from build123d import *

# Parameters (mm, degrees)
F1_DEPTH = 11
F2_DEPTH = 4


with BuildPart() as f1:
    # F0 (on Top) → F1 (new body)
    with BuildSketch(Plane.XY):
        with BuildLine():
            ThreePointArc((94, 77.5), (93.267767, 79.267767), (91.5, 80))
            Line((91.5, 80), (40.553054, 80))
            Line((40.553054, 80), (23, 80))
            Line((23, 80), (17.5, 80))
            Line((17.5, 80), (-7.5, 80))
            Line((-7.5, 80), (-13, 80))
            Line((-13, 80), (-32.2531, 80))
            Line((-32.2531, 80), (-74.5, 80))
            Line((-74.5, 80), (-91.5, 80))
            ThreePointArc((-91.5, 80), (-93.267767, 79.267767), (-94, 77.5))
            Line((-94, 77.5), (-94, 76))
            Line((-94, 76), (-94, 0))
            Line((-94, 0), (-94, -1.5))
            ThreePointArc((-94, -1.5), (-93.267767, -3.267767), (-91.5, -4))
            Line((-91.5, -4), (-88, -4))
            Line((-88, -4), (88, -4))
            Line((88, -4), (91.5, -4))
            ThreePointArc((91.5, -4), (93.267767, -3.267767), (94, -1.5))
            Line((94, -1.5), (94, 0))
            Line((94, 0), (94, 76))
            Line((94, 76), (94, 77.5))
        make_face()
        with BuildLine():
            ThreePointArc((90, 2.5), (89.267767, 0.732233), (87.5, 0))
            Line((87.5, 0), (-87.5, 0))
            ThreePointArc((-87.5, 0), (-89.267767, 0.732233), (-90, 2.5))
            Line((-90, 2.5), (-90, 73.5))
            ThreePointArc((-90, 73.5), (-89.267767, 75.267767), (-87.5, 76))
            Line((-87.5, 76), (87.5, 76))
            ThreePointArc((87.5, 76), (89.267767, 75.267767), (90, 73.5))
            Line((90, 73.5), (90, 2.5))
        make_face(mode=Mode.SUBTRACT)
    extrude(amount=F1_DEPTH)

    # F0 (on Top) → F2 (join)
    with BuildSketch(Plane.XY):
        with BuildLine():
            Line((-87.5, 0), (87.5, 0))
            ThreePointArc((87.5, 0), (89.267767, 0.732233), (90, 2.5))
            Line((90, 2.5), (90, 73.5))
            ThreePointArc((90, 73.5), (89.267767, 75.267767), (87.5, 76))
            Line((87.5, 76), (-87.5, 76))
            ThreePointArc((-87.5, 76), (-89.267767, 75.267767), (-90, 73.5))
            Line((-90, 73.5), (-90, 2.5))
            ThreePointArc((-90, 2.5), (-89.267767, 0.732233), (-87.5, 0))
        make_face()
        with BuildLine():
            Line((-77.5, 66), (77.5, 66))
            ThreePointArc((77.5, 66), (79.267767, 65.267767), (80, 63.5))
            Line((80, 63.5), (80, 12.5))
            ThreePointArc((80, 12.5), (79.267767, 10.732233), (77.5, 10))
            Line((77.5, 10), (-77.5, 10))
            ThreePointArc((-77.5, 10), (-79.267767, 10.732233), (-80, 12.5))
            Line((-80, 12.5), (-80, 63.5))
            ThreePointArc((-80, 63.5), (-79.267767, 65.267767), (-77.5, 66))
        make_face(mode=Mode.SUBTRACT)
        with BuildLine():
            Line((-32.2531, 80), (-13, 80))
            Line((-13, 80), (-13, 89.5))
            ThreePointArc((-13, 89.5), (-13.732233, 91.267767), (-15.5, 92))
            Line((-15.5, 92), (-29.7531, 92))
            ThreePointArc((-29.7531, 92), (-31.520867, 91.267767), (-32.2531, 89.5))
            Line((-32.2531, 89.5), (-32.2531, 80))
        make_face()
        with BuildLine():
            Line((-7.5, 80), (17.5, 80))
            Line((17.5, 80), (17.5, 89.5))
            ThreePointArc((17.5, 89.5), (16.767767, 91.267767), (15, 92))
            Line((15, 92), (-5, 92))
            ThreePointArc((-5, 92), (-6.767767, 91.267767), (-7.5, 89.5))
            Line((-7.5, 89.5), (-7.5, 80))
        make_face()
        with BuildLine():
            Line((23, 80), (40.553054, 80))
            Line((40.553054, 80), (40.553054, 90.5))
            ThreePointArc((40.553054, 90.5), (39.820821, 92.267767), (38.053054, 93))
            Line((38.053054, 93), (25.5, 93))
            ThreePointArc((25.5, 93), (23.732233, 92.267767), (23, 90.5))
            Line((23, 90.5), (23, 80))
        make_face()
    extrude(amount=F2_DEPTH)


solid = f1.part
Part model, mm, in its own coordinate system. A direction names the side the tool comes from. Coordinates: 2 decimals unless noted, no trailing zeros. Loops run counter-clockwise (first coordinate to the right, second up) from the corner with the lowest first, then second, coordinate; pieces in that order, holes last. Notation, with made-up numbers: (7.5, -6) - (55.5, -6) arc R20 cw to (55.5, 17) - close; hole circle Ø9 at (49.25, -28). An arc over 180 degrees is marked (long way). Write each question's results on one line, items separated by ' | '. Start each with the question number.
Q1. Two-plate mould, pull along X, no slides. Class faces 4 (the flat face through (-1, 66, 2)), 5 (the flat face through (-94, 39, 5)), 6 (the flat face through (-23, 92, 2)), 7 (the flat face through (94, 37, 5)): +X half, -X half, draft (parallel to the pull), parting line (faces both ways), or undercut.
Q2. Slice it at B-B on y = 82. Give the cut face in (x, z).
Q3. Which spindle directions (+Z, -Z, +X, -X, +Y, -Y) get a long thin tool onto all of the face, cutting with end or side? Do faces 1 (the flat face through (5, 92, 2)), 2 (the flat face through (40.553, 85, 2)), 3 (the flat face through (-1, 76, 7)). Say none if no direction does.
Q4. Drop flat-ended pins along their axis: pin 1 Ø2 at (x, z) = (14.5, 2) entering from +Y; pin 2 Ø2 at (y, z) = (83, 1.5) entering from +X; pin 3 Ø10.5 at (x, y) = (31.5, 86.5) entering from +Z. Give the stop position or say it passes through.
Q5. Probe line 1 along X through (y, z) = (29, 1.5); line 2 along Y through (x, z) = (62, 8.75); line 3 along X through (y, z) = (12, 6.25). List the from-to ranges inside material, lowest first.
Q6. Slice it at D-D on z = 8. Give the cut face in (x, y), and give its area (3 significant figures).
Q7. Slice it at C-C on x = 62. Give the cut face in (y, z), and give its area (3 significant figures).
Q8. Slice it at A-A on y = 43.5. Give the cut face in (x, z).
Answer:
1) face 4: undercut | face 5: -X half | face 6: draft | face 7: +X half
2) outline: (-32.25, 0) - (-13, 0) - (-13, 4) - (-32.25, 4) - close; (-7.5, 0) - (17.5, 0) - (17.5, 4) - (-7.5, 4) - close; (23, 0) - (40.55, 0) - (40.55, 4) - (23, 4) - close
3) face 1: +Z, -Z, -X, +Y | face 2: +Z, -Z, +X, +Y | face 3: +Z
4) pin 1: stops at y = 92 | pin 2: stops at x = 40.55 | pin 3: stops at z = 4
5) line 1: x = -94 to -80, 80 to 94 | line 2: y = -4 to 0, 76 to 80 | line 3: x = -94 to -90, 90 to 94
6) outline: (-94, -1.5) arc R2.5 ccw to (-91.5, -4) - (91.5, -4) arc R2.5 ccw to (94, -1.5) - (94, 77.5) arc R2.5 ccw to (91.5, 80) - (-91.5, 80) arc R2.5 ccw to (-94, 77.5) - close; hole (-90, 2.5) arc R2.5 ccw to (-87.5, 0) - (87.5, 0) arc R2.5 ccw to (90, 2.5) - (90, 73.5) arc R2.5 ccw to (87.5, 76) - (-87.5, 76) arc R2.5 ccw to (-90, 73.5) - close | area: 2,110 mm2
7) outline: (-4, 0) - (10, 0) - (10, 4) - (0, 4) - (0, 11) - (-4, 11) - close; (66, 0) - (80, 0) - (80, 11) - (76, 11) - (76, 4) - (66, 4) - close | area: 168 mm2
8) outline: (-94, 0) - (-80, 0) - (-80, 4) - (-90, 4) - (-90, 11) - (-94, 11) - close; (80, 0) - (94, 0) - (94, 11) - (90, 11) - (90, 4) - (80, 4) - close
